The listing builds one solid part. Answer for the finished solid, in the listing's coordinates (mm). A direction names the side the tool comes from. Coordinates: 2 decimals unless noted, no trailing zeros. Order: outer loops, then holes, each group sorted by start corner. A loop starts at its lowest first (then second) coordinate and runs counter-clockwise, first axis right, second up. Notation, with made-up numbers: (-2.75, 84.25) -> (38.25, 84.25) arc R31 ccw to (38.25, 121.25) -> close; hole circle Ø9 at (-10, -40). An arc over 180 degrees is marked (long way). Return JSON: item names as keys, results as strings.
from build123d import *

# Parameters (mm, degrees)
F0_R      = 2
F1_DEPTH  = 4
F3_DEPTH  = 2
F5_DEPTH  = 50
F7_DEPTH  = 8
F9_DEPTH  = 8
F10_W     = 22.2
F10_H     = 36
F11_DEPTH = 60


with BuildPart() as f1:
    # F0 (on Top) → F1 (new body)
    with BuildSketch(Plane.XY):
        Polygon((26.85, 17.5), (-26.85, 17.5), (-26.85, 32.5), (-29, 32.5), (-29, 17.5), (-29, -17.5), (29, -17.5), (29, 17.5), (29, 32.5), (26.85, 32.5), align=None)
        with Locations((0, -9.5)):
            Circle(F0_R, mode=Mode.SUBTRACT)
        with Locations((-21, 9.5)):
            Circle(F0_R, mode=Mode.SUBTRACT)
        with Locations((21, 9.5)):
            Circle(F0_R, mode=Mode.SUBTRACT)
    extrude(amount=F1_DEPTH)

    # F2 (on face) → F3 (join)
    with BuildSketch(Plane.XY.offset(4)):
        Polygon((26.85, 32.5), (26.85, 17.5), (-26.85, 17.5), (-26.85, 32.5), (-29, 32.5), (-29, -17.5), (29, -17.5), (29, 32.5), align=None)
        Polygon((3.05, -11.260918321), (0, -13.0218366421), (-3.05, -11.260918321), (-3.05, -7.739081679), (0, -5.9781633579), (3.05, -7.739081679), align=None, mode=Mode.SUBTRACT)
        Polygon((-17.4781633579, 9.5), (-19.239081679, 6.45), (-22.760918321, 6.45), (-24.5218366421, 9.5), (-22.760918321, 12.55), (-19.239081679, 12.55), align=None, mode=Mode.SUBTRACT)
        Polygon((22.760918321, 12.55), (24.5218366421, 9.5), (22.760918321, 6.45), (19.239081679, 6.45), (17.4781633579, 9.5), (19.239081679, 12.55), align=None, mode=Mode.SUBTRACT)
    extrude(amount=F3_DEPTH)

    # F4 (on face) → F5 (join)
    with BuildSketch(Plane.XY.offset(6)):
        Polygon((-25.5, 3.5), (-25.5, 17.5), (-26.85, 17.5), (-26.85, 32.5), (-29, 32.5), (-29, -17.5), (29, -17.5), (29, 32.5), (26.85, 32.5), (26.85, 17.5), (25.5, 17.5), (25.5, 3.5), (22, 3.5), (22, -14.5), (-22, -14.5), (-22, 3.5), align=None)
    extrude(amount=F5_DEPTH)

    # F6 (on face) → F7 (cut)
    with BuildSketch(Plane(origin=(-29, 0, 0), x_dir=(0, -1, 0), z_dir=(-1, 0, 0))):
        with BuildLine():
            Line((0.7, 56), (0.7, 13.6))
            ThreePointArc((0.7, 13.6), (6.7, 7.6), (12.7, 13.6))
            Line((12.7, 13.6), (12.7, 56))
            Line((12.7, 56), (0.7, 56))
        make_face()
    extrude(amount=-F7_DEPTH, mode=Mode.SUBTRACT)

    # F8 (on face) → F9 (cut)
    with BuildSketch(Plane.YZ.offset(29)):
        with BuildLine():
            Line((-12.7, 56), (-12.7, 16.2))
            ThreePointArc((-12.7, 16.2), (-6.7, 10.2), (-0.7, 16.2))
            Line((-0.7, 16.2), (-0.7, 56))
            Line((-0.7, 56), (-12.7, 56))
        make_face()
    extrude(amount=-F9_DEPTH, mode=Mode.SUBTRACT)

    # F10 (on face) → F11 (cut)
    with BuildSketch(Plane.YZ.offset(29)):
        with Locations((21.4, 38)):
            Rectangle(F10_W, F10_H)
    extrude(amount=-F11_DEPTH, mode=Mode.SUBTRACT)


solid = f1.part
1. For faces 3 (the face through (26, -12.7, 36)), 4 (the face through (23.654, 7.996, 4.986)), 5 (the face through (25.5, 9, 25)), 6 (the face through (-22.474, 10.852, 1.972)), 7 (the face through (-27, 10.3, 38)), determine the directions among +Z, -Z, +X, -X, +Y, -Y from which every point of the face is accessible in a straight line to the end or side of a thin tool.
Answer block:
{"face 3": "+Z, +X, -X", "face 4": "+Z", "face 5": "+Z, +Y", "face 6": "+Z, -Z", "face 7": "+Z, +X, -X, +Y"}
2. The part is cut by section B-B on x = -21. Give the vertices of the cut face in (y, z).
Answer block:
{"outline": "(-17.5, 0) -> (7.5, 0) -> (7.5, 4) -> (6.45, 4) -> (6.45, 6) -> (-14.5, 6) -> (-14.5, 56) -> (-17.5, 56) -> close; (11.5, 0) -> (17.5, 0) -> (17.5, 6) -> (12.55, 6) -> (12.55, 4) -> (11.5, 4) -> close"}
3. Consider line 1 (X direction, y = 2.5, z = 45); line 2 (Y direction, x = 0, z = 3); line 3 (Y direction, x = 21, z = 1.1). Determine where each line is inside the solid, lowest interval first. Write a range as from..to.
Answer block:
{"line 1": "x = -29..-22, 22..29", "line 2": "y = -17.5..-11.5, -7.5..17.5", "line 3": "y = -17.5..7.5, 11.5..17.5"}
4. Each of these flat-tipped pins is pushed along its axis until it touches: pin 1 Ø1.8 at (x, z) = (26.5, 34.5) entering from +Y; pin 2 Ø3 at (x, y) = (-27, 16) entering from +Z; pin 3 Ø22 at (x, z) = (-10, 35) entering from +Y. Where does it stop, or does it pass through?
Answer block:
{"pin 1": "stops at y = 10.3", "pin 2": "stops at z = 20", "pin 3": "stops at y = -14.5"}
5. The part is cut by section D-D on y = -9.5. Give the vertices of the cut face in (x, z), and give its area (3 significant figures).
Answer block:
{"outline": "(-29, 0) -> (-2, 0) -> (-2, 4) -> (-3.05, 4) -> (-3.05, 6) -> (-22, 6) -> (-22, 8.29) -> (-29, 8.29) -> close; (2, 0) -> (29, 0) -> (29, 10.89) -> (22, 10.89) -> (22, 6) -> (3.05, 6) -> (3.05, 4) -> (2, 4) -> close", "area": "370 mm2"}
6. The part is cut by section A-A on z = 48. Give the vertices of the cut face in (x, y).
Answer block:
{"outline": "(-29, -17.5) -> (29, -17.5) -> (29, -12.7) -> (22, -12.7) -> (22, -14.5) -> (-22, -14.5) -> (-22, -12.7) -> (-29, -12.7) -> close; (-29, -0.7) -> (-22, -0.7) -> (-22, 3.5) -> (-25.5, 3.5) -> (-25.5, 10.3) -> (-29, 10.3) -> close; (22, -0.7) -> (29, -0.7) -> (29, 10.3) -> (25.5, 10.3) -> (25.5, 3.5) -> (22, 3.5) -> close"}
7. The part is cut by section C-C on y = 16.5. Give the vertices of the cut face in (x, z).
Answer block:
{"outline": "(-29, 0) -> (29, 0) -> (29, 20) -> (25.5, 20) -> (25.5, 6) -> (-25.5, 6) -> (-25.5, 20) -> (-29, 20) -> close"}
8. Determine the mould class of faces 1 (the face through (-25.5, 9, 25)), 2 (the face through (0, -16, 56)) for opening direction X: pulls with the +X half, pulls with the -X half, needs draft (parallel to the pull), parting line crosses it, or undercut.
Answer block:
{"face 1": "undercut", "face 2": "needs draft"}
